Autodesk Inventor part; units mm, degrees
ref_plane "YZ Plane" through (0, 0, 0) normal (1, 0, 0) x (0, 1, 0)
ref_plane "XZ Plane" through (0, 0, 0) normal (0, 1, 0) x (-1, 0, 0)
ref_plane "XY Plane" through (0, 0, 0) normal (0, 0, 1) x (1, 0, 0)
sketch "Sketch1" plane through (0, 0, 0) normal (0, 0, 1) x (1, 0, 0)
  line L0 (-1.1769, 0) -> (22.352, 0)
  line L1 (22.352, 0) -> (22.352, 3.9687)
  line L2 (22.352, 3.9687) -> (9.652, 3.9687)
  line L3 (9.652, 3.9687) -> (9.652, 4.7371)
  line L4 (9.652, 4.7371) -> (0, 4.7371)
  line L5 (0, 4.7371) -> (0, 7.1374)
  line L6 (0, 7.1374) -> (-6.35, 7.1374)
  line L7 (-6.35, 7.1374) -> (-6.35, 2.757)
  line L8 (-6.35, 2.757) -> (-2.7686, 2.757)
  line L9 (-2.7686, 2.757) -> (-1.1769, 0)
  line L10 (-12.0904, 0) -> (28.0924, 0)
  line L11 (0, -1.4275) -> (0, 8.5649)
  line L12 (0, 4.4704) -> (2.0955, 4.4704)
  line L13 (2.0955, 4.4704) -> (2.3622, 4.7371)
  line L14 (9.652, 3.9687) -> (9.652, 3.1293)
  line L15 (9.652, 3.1293) -> (12.4714, 3.1293)
  line L16 (12.4714, 3.1293) -> (13.3109, 3.9687)
  line L17 (0, 4.4704) -> (0, 4.7371)
  dimension "d0" = 7.9375
  dimension "d1" = 9.4742
  dimension "d2" = 14.2748
  dimension "d3" = 5.5139
  dimension "d5" = 12.7
  dimension "d6" = 6.35
  dimension "d7" = 3.5814
  dimension "d8" = 60
  dimension "d9" = 22.352
  dimension "d19" = 45
  dimension "d20" = 8.9408
  dimension "d21" = 6.2586
  dimension "d22" = 45
  dimension "d23" = 2.8194
  dimension "d34" = 2.3622
revolve "Body" add sketch "Sketch1" angle 360 about axis through (-1.1769, 0, 0) along (1, 0, 0)
sketch "Sketch2" plane through (-6.35, 0, 0) normal (-1, 0, 0) x (0, 0, 1)
  circle A0 centre (0, 0) radius 2.757
  line L0 (0, 2.757) -> (2.3876, 1.3785)
  line L1 (2.3876, 1.3785) -> (2.3876, -1.3785)
  line L2 (2.3876, -1.3785) -> (0, -2.757)
  line L3 (0, -2.757) -> (-2.3876, -1.3785)
  line L4 (-2.3876, -1.3785) -> (-2.3876, 1.3785)
  line L5 (-2.3876, 1.3785) -> (0, 2.757)
extrude "Slot" add sketch "Sketch2" against normal up to next contours A0 L1 | L0 A0 | A0 L2 | L5 A0 | A0 L3 | L4 A0
fillet "Fillet1" radius 2.3622 1 edges at (-6.35, -7.1374, 0)
thread "Thread"
chamfer "Chamfer1" distance 0.8395 distance2 0.8395 1 edges at (22.352, -3.9687, 0) measured on face at (22.352, 0.1595, 1.1606)
chamfer "Chamfer2" distance 0.127 angle 45 1 edges at (9.652, -4.7371, 0) measured on face at (9.652, 4.3967, -0.6945)
revolve "Groove1" cut sketch "Sketch1" angle 360 about axis through (-1.1769, 0, 0) along (1, 0, 0) contours L11 L4 L13 L12
revolve "Groove2" cut sketch "Sketch1" angle 360 about axis through (-1.1769, 0, 0) along (1, 0, 0) contours L16 L15 L14 L2
equation "\"d0\" = NND"
equation "\"d1\" = BDM"
equation "\"d2\" = KOD"
equation "\"d3\" = 1.1547 * SW"
equation "\"d5\" = GEL"
equation "\"d6\" = KOH"
equation "\"d7\" = INTI + LOTI"
equation "\"d8\" = 0.5 * ANG"
equation "\"d9\" = NLG"
equation "\"d19\" = FAWI4"
equation "\"d20\" = BDMM"
equation "\"d21\" = GD1"
equation "\"d22\" = FAWI2"
equation "\"d23\" = GAL"
equation "\"d34\" = GAL2"
equation "\"d13\" = RR"
equation "\"d25\" = GEL"
equation "\"d14\" = -0.5 * SPD + 0.5 * NND"
equation "\"d15\" = GUL"
equation "\"d32\" = -0.5 * NND + 0.5 * BDM"
equation "\"NND\" = 7.9375"
equation "\"NLG\" = 22.352"
equation "\"GEL\" = 12.7"
equation "\"KOD\" = 14.2748"
equation "\"KOH\" = 6.35"
equation "\"INTI\" = 3.5814"
equation "\"GAL\" = 2.8194"
equation "\"GUL\" = 0.83947"
equation "\"SPD\" = GD1"
equation "\"BDM\" = 9.4742"
equation "\"ANG\" = 120deg"
equation "\"FAWI2\" = 45deg"
equation "\"FAWI3\" = 45deg"
equation "\"FAWI4\" = 45deg"
equation "\"RR\" = 2.3622"
equation "\"SW\" = 4.7752"
equation "\"BDMM\" = 8.9408"
equation "\"GAL2\" = RR"
equation "\"LOTI\" = 0"
equation "\"GD1\" = 6.25856"
equation "\"BOR\" = SW"
equation "\"SLG\" = 9.652"
equation "\"THREADDIA\" = 7.9375"
equation "\"E0\" = 1.155 * SW"
equation "\"FAWI1\" = 45deg"
equation "\"TOA\" = 30deg"
equation "\"PHH\" = RR"
equation "\"HHPTC\" = 1.41122"
equation "\"GD0\" = 6.0198"
equation "\"KOH1\" = 5.3086"
equation "\"BDMN\" = 9.525"
properties part number "ANSI B18.3 - 0.375 x 0.38 ANSI B18.3" material "Steel, Mild"
Geometry: final body of the model. Coordinates: model frame, mm. A direction names the side the tool comes from. Give positions to 0.01 mm unless a question says otherwise; leave off trailing zeros. Write each loop counter-clockwise with the first axis right and the second up, starting at its lowest first coordinate (ties: lowest second). Pieces come first, ordered by that corner, then holes. Notation, with made-up numbers: (-14, -3) - (-8, -3) arc R11 ccw to (-8, 4) - close; hole circle Ø8 at (44.25, 21). An arc over 180 degrees is marked (long way). Return JSON: item names as keys, results as strings. Group by question number.
1) Set-up query: faces 1 (the flat face through (-6.35, -2, 2)), 2 (the cylindrical face through (11.081, -0.678, -3.055)), 3 (the flat face through (-4, 0, -2.388)). Return all of +Z, -Z, +X, -X, +Y, -Y with unobstructed straight access to the full face (end or side cutting, diameter ignored); none if empty.
2) First-contact query: P1, Ø2, axis at x = 11.5, z = -1, coming from the -Y side; P2, Ø5, axis at x = 2, z = 3, coming from the +Y side; P3, Ø1.5, axis at x = -3, y = -5, coming from the -Z side. Flat tips, straight axial feed; report the tip coordinate or a pass-through.
3) Mould query, pull axis Z, two halves, no side actions, for faces 4 (the flat face through (-4.48, -2.06, 1.21)), 5 (the cylindrical face through (17.354, -0.86, 3.874)), 6 (the flat face through (0, 0, -5)). Classes: released by +Z, released by -Z, zero draft, split by the parting line, or undercut.
4) Section B-B on x = 2.75. Return the cut outline in (y, z), plus the area to 3 significant figures.
5) Section A-A on x = 17. Return the cut outline in (y, z).
6) Line query: line 1 (Y direction, x = -3.25, z = 1.5); line 2 (X direction, y = -4.75, z = 1.25); line 3 (Z direction, x = -1.25, y = -1). Output: solid intervals per line, ascending.
Filled in:
{
 "1": {"face 1": "+Z, -Z, -X, +Y, -Y", "face 2": "none", "face 3": "-X"},
 "2": {"P1": "stops at y = -3.13", "P2": "stops at y = 6.98", "P3": "stops at z = -5.73"},
 "3": {"face 4": "undercut", "face 5": "split by the parting line", "face 6": "zero draft"},
 "4": {"outline": "circle Ø9.47 at (0, 0)", "area": "70.5 mm^2"},
 "5": {"outline": "circle Ø7.94 at (0, 0)"},
 "6": {"line 1": "y = -6.98 to -1.89, 1.89 to 6.98", "line 2": "x = -6.35 to 0", "line 3": "z = -7.07 to 7.07"}
}
